Autodesk Inventor part; units mm, degrees
ref_plane "YZ Plane" through (0, 0, 0) normal (1, 0, 0) x (0, 1, 0)
ref_plane "XZ Plane" through (0, 0, 0) normal (0, 1, 0) x (-1, 0, 0)
ref_plane "XY Plane" through (0, 0, 0) normal (0, 0, 1) x (1, 0, 0)
sketch "Sketch1" plane through (0, 0, 0) normal (0, 1, 0) x (-1, 0, 0)
  line L0 (125, 50) -> (-125, 50)
  line L1 (-125, 50) -> (-125, -50)
  line L2 (-125, -50) -> (125, -50)
  line L3 (125, -50) -> (125, 50)
  line L4 (120, 45) -> (-120, 45)
  line L5 (-120, 45) -> (-120, -45)
  line L6 (-120, -45) -> (120, -45)
  line L7 (120, -45) -> (120, 45)
  point P0 (0, 0)
  dimension "d0" = 250
  dimension "d1" = 100
  dimension "d2" = 50
  dimension "d3" = 125
  dimension "d4" = 5
  dimension "d5" = 5
  dimension "d6" = 5
  dimension "d7" = 5
extrude "Extrusion1" add sketch "Sketch1" along normal blind 5 contours L7 L6 L5 L4
sketch "Sketch2" plane through (0, 0, 0) normal (0, -1, 0) x (1, 0, 0)
  line L0 (-125, -50) -> (125, -50)
  line L1 (125, -50) -> (125, 50)
  line L2 (125, 50) -> (-125, 50)
  line L3 (-125, 50) -> (-125, -50)
  line L4 (-120, -45) -> (-120, 45)
  line L5 (120, 45) -> (120, -45)
  line L6 (-120, 45) -> (120, 45)
  line L7 (120, -45) -> (-120, -45)
  line L8 (-120, -45) -> (-120, 45)
  line L9 (120, 45) -> (120, -45)
  line L10 (-120, -45) -> (120, -45)
  line L11 (120, -45) -> (120, 45)
  line L12 (120, 45) -> (-120, 45)
  line L13 (-120, 45) -> (-120, -45)
  point P0 (0, 0)
  dimension "d10" = 5
  dimension "d11" = 5
  dimension "d12" = 5
  dimension "d13" = 5
extrude "Extrusion2" add sketch "Sketch2" against normal blind 120
sketch "Sketch4" plane through (-125, 0, 50) normal (0, 0, 1) x (1, 0, 0)
  circle A0 centre (65, 70) radius 2.5
  circle A1 centre (185, 70) radius 2.5
  line L0 (250, 0) -> (0, 0)
  line L1 (250, 0) -> (250, 120)
  point P0 (125, 0)
  point P1 (250, 60)
  dimension "d16" = 5
  dimension "d17" = 5
  dimension "d18" = 70
  dimension "d19" = 70
  dimension "d20" = 120
  dimension "d21" = 65
extrude "Extrusion3" cut sketch "Sketch4" against normal blind 5
properties part number "Team29_BaseofBox"
Here's how the part is built. I have some questions about the finished solid (model axes, mm). A direction names the side the tool comes from. Give positions to 0.01 mm unless a question says otherwise; leave off trailing zeros. Order: outer loops, then holes, each group sorted by start corner. A loop starts at its lowest first (then second) coordinate and runs counter-clockwise, first axis right, second up. Notation, with made-up numbers: (-33, 32) -> (17, 32) arc R28 cw to (17, 64) -> close; hole circle Ø1 at (60, 67). An arc over 180 degrees is marked (long way). Use a Markdown table: item, result. Add a question column.
Item 1: For faces 1 (the face through (-38, 120, -48)), 2 (the face through (-120, 62, -1)), 3 (the face through (-57.69, 69.04, 47.54)), which set-ups out of +Z, -Z, +X, -X, +Y, -Y let a thin tool reach every point of the face, with its end or its side?
Item 2: Will this pin go through, and if not, where does the flat tip stop? pin 1 (5 mm diameter, centred on x = -21, z = -29, fed in from +Y).
Item 3: Imagine slicing it at B-B on x = -60. Please give me the cut outline in (y, z).
Item 4: Imagine slicing it at C-C on z = 13.5. Please give me the cut outline in (x, y), plus the area to 3 significant figures.
Item 5: Imagine slicing it at A-A on y = 70. Please give me the cut outline in (x, z), plus the area to 3 significant figures.
Item 6: Imagine slicing it at D-D on y = 105.5. Please give me the cut outline in (x, z).
Item 7: If we mould it in two halves opening along Z, with no side actions, what happens to faces 4 (the face through (-2, 59, -50)), 5 (the face through (-2, 62, 45)), 6 (the face through (2, 59, 50)), 7 (the face through (2, 0, 1))? For each: pulls with the +Z half, pulls with the -Z half, needs draft (parallel to the pull), parting line crosses it, or undercut.
Item 8: I need wall thicknesses on line 1 (X direction, y = 29, z = 25.5); line 2 (Y direction, x = 60, z = 48); line 3 (Z direction, x = -110, y = 87). Which ranges of each line are inside material? Lowest first, please.
Data:
| question | item | result |
|---|---|---|
| 1 | face 1 | +Z, -Z, +X, -X, +Y |
| 1 | face 2 | +Y |
| 1 | face 3 | +Z |
| 2 | pin 1 | stops at y = 5 |
| 3 | outline | (0, -50) -> (120, -50) -> (120, -45) -> (5, -45) -> (5, 45) -> (67.5, 45) -> (67.5, 50) -> (0, 50) -> close; (72.5, 45) -> (120, 45) -> (120, 50) -> (72.5, 50) -> close |
| 4 | outline | (-125, 0) -> (125, 0) -> (125, 120) -> (120, 120) -> (120, 5) -> (-120, 5) -> (-120, 120) -> (-125, 120) -> close |
| 4 | area | 2,400 mm² |
| 5 | outline | (-125, -50) -> (125, -50) -> (125, 50) -> (62.5, 50) -> (62.5, 45) -> (120, 45) -> (120, -45) -> (-120, -45) -> (-120, 45) -> (-62.5, 45) -> (-62.5, 50) -> (-125, 50) -> close; (-57.5, 45) -> (57.5, 45) -> (57.5, 50) -> (-57.5, 50) -> close |
| 5 | area | 3,350 mm² |
| 6 | outline | (-125, -50) -> (125, -50) -> (125, 50) -> (-125, 50) -> close; hole (-120, -45) -> (120, -45) -> (120, 45) -> (-120, 45) -> close |
| 7 | face 4 | pulls with the -Z half |
| 7 | face 5 | undercut |
| 7 | face 6 | pulls with the +Z half |
| 7 | face 7 | needs draft |
| 8 | line 1 | x = -125 to -120, 120 to 125 |
| 8 | line 2 | y = 0 to 67.5, 72.5 to 120 |
| 8 | line 3 | z = -50 to -45, 45 to 50 |
